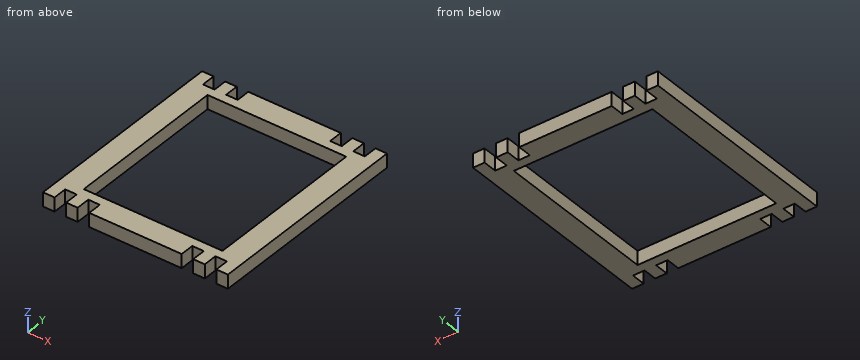
Autodesk Fusion 360 part; units mm, degrees
sketch "Sketch1" plane through (0, 0, 0) normal (0, 0, 1) x (1, 0, 0)
  line L0 (40, 45) -> (-40, 45)
  line L1 (-40, 45) -> (-40, -45)
  line L2 (-40, -45) -> (40, -45)
  line L3 (40, -45) -> (40, 45)
  line L4 (40, 45) -> (-40, -45) construction
  line L5 (-40, 45) -> (40, -45) construction
  line L6 (30, 35) -> (-30, 35)
  line L7 (-30, 35) -> (-30, -35)
  line L8 (-30, -35) -> (30, -35)
  line L9 (30, -35) -> (30, 35)
  line L10 (30, 35) -> (-30, -35) construction
  line L11 (-30, 35) -> (30, -35) construction
  dimension "d1" = 80
  dimension "d2" = 90
  dimension "d3" = 60
  dimension "d6" = 10
extrude "Extrude1" add sketch "Sketch1" along normal blind 6
sketch "Sketch2" plane through (0, 0, 6) normal (0, 0, 1) x (-1, 0, 0)
  line L0 (-30, -35) -> (-30, 35)
  line L1 (-30, 35) -> (30, 35)
  line L2 (30, 35) -> (30, -35)
  line L3 (30, -35) -> (-30, -35)
  line L4 (-40, 45) -> (-40, -45)
  line L5 (-40, -45) -> (40, -45)
  line L6 (40, -45) -> (40, 45)
  line L7 (40, 45) -> (-40, 45)
  line L8 (-40, 45) -> (-35, 45) construction
  line L9 (-35, 45) -> (-35, 39) construction
  line L10 (-35, 39) -> (-40, 39) construction
  line L11 (-40, 39) -> (-40, 45) construction
  line L12 (-35, 45) -> (-30, 45) construction
  line L13 (-30, 45) -> (-30, 39) construction
  line L14 (-30, 39) -> (-35, 39) construction
  line L15 (-35, 39) -> (-35, 45) construction
  line L16 (-30, 45) -> (-25, 45) construction
  line L17 (-25, 45) -> (-25, 39) construction
  line L18 (-25, 39) -> (-30, 39) construction
  line L19 (-30, 39) -> (-30, 45) construction
  line L20 (-25, 45) -> (-20, 45) construction
  line L21 (-20, 45) -> (-20, 39) construction
  line L22 (-20, 39) -> (-25, 39) construction
  line L23 (-25, 39) -> (-25, 45) construction
  line L24 (-30, 39) -> (-35, 39)
  line L25 (-35, 39) -> (-35, 45)
  line L26 (-35, 45) -> (-30, 45)
  line L27 (-30, 45) -> (-30, 39)
  line L28 (-20, 39) -> (-25, 39)
  line L29 (-25, 39) -> (-25, 45)
  line L30 (-25, 45) -> (-20, 45)
  line L31 (-20, 45) -> (-20, 39)
  line L32 (40, 45) -> (35, 45) construction
  line L33 (35, 45) -> (35, 39) construction
  line L34 (35, 39) -> (40, 39) construction
  line L35 (40, 39) -> (40, 45) construction
  line L36 (35, 39) -> (30, 39)
  line L37 (30, 39) -> (30, 45)
  line L38 (30, 45) -> (35, 45)
  line L39 (35, 45) -> (35, 39)
  line L40 (30, 39) -> (25, 39) construction
  line L41 (25, 39) -> (25, 45) construction
  line L42 (25, 45) -> (30, 45) construction
  line L43 (30, 45) -> (30, 39) construction
  line L44 (25, 39) -> (20, 39)
  line L45 (20, 39) -> (20, 45)
  line L46 (20, 45) -> (25, 45)
  line L47 (25, 45) -> (25, 39)
extrude "Extrude2" cut sketch "Sketch2" against normal blind 6 contours L7 L24 L25 L26 L27 | L7 L28 L29 L30 L31
ref_plane "WorkPlane1" through (0, 0, 0) normal (0, 1, 0) x (0, 0, 1)
ref_plane "WorkPlane2" through (0, 0, 0) normal (1, 0, 0) x (0, 1, 0)
extrude "Extrude3" cut sketch "Sketch2" against normal blind 6 contours L7 L24 L25 L26 L27 | L7 L28 L29 L30 L31 | L7 L36 L37 L38 L39 | L7 L44 L45 L46 L47
mirror "Mirror3" about plane through (0, 0, 0) normal (0, 1, 0) of "Extrude3"
The listing builds one solid part. Answer for the finished solid, in the listing's coordinates (mm). Give positions to 0.01 mm unless a question says otherwise; leave off trailing zeros. Loops run counter-clockwise (first coordinate to the right, second up) from the corner with the lowest first, then second, coordinate; pieces in that order, holes last. Notation, with made-up numbers: (-37, 76.25) - (14, 76.25) arc R35 ccw to (14, 109.25) - close; hole circle Ø6 at (-8, 34). An arc over 180 degrees is marked (long way). Answer as a JSON object with one key per item and string values.
1. Find the intervals of material crossed by L1, parallel to Y at x = -25.5, z = 4.75; L2, parallel to X at y = 28.5, z = 1.2; L3, parallel to Y at x = -34.5, z = 1.7, in increasing order. Write a range as [from, to].
Determined:
{"L1": "[-45, -35], [35, 45]", "L2": "[-40, -30], [30, 40]", "L3": "[-39, 39]"}
2. A cutting plane is placed at A-A (x = 17). Write down the section's boundary in (y, z), then the cut area to 3 significant figures.
Determined:
{"outline": "(-45, 0) - (-35, 0) - (-35, 6) - (-45, 6) - close; (35, 0) - (45, 0) - (45, 6) - (35, 6) - close", "area": "120 mm²"}
3. Flat-ended cylindrical pins translate along their axes: pin 1 Ø2.5 at (x, z) = (-33.5, 2.5) entering from +Y; pin 2 Ø2.5 at (x, z) = (-22.5, 2) entering from -Y. Find the tip coordinate at first contact, or state that the pin passes through.
Determined:
{"pin 1": "y = 39", "pin 2": "y = -39"}
4. A cutting plane is placed at B-B (y = -20). Write down the section's boundary in (x, z), then the cut area to 3 significant figures.
Determined:
{"outline": "(-40, 0) - (-30, 0) - (-30, 6) - (-40, 6) - close; (30, 0) - (40, 0) - (40, 6) - (30, 6) - close", "area": "120 mm²"}
